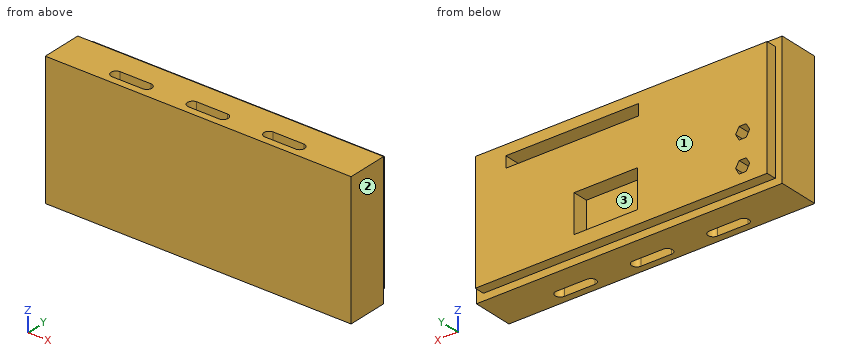
```python
from build123d import *

# Parameters (mm, degrees)
SKETCH1_W           = 150
SKETCH1_H           = 65
BOSS_EXTRUDE1_DEPTH = 20
CUT_EXTRUDE1_DEPTH  = 66
SKETCH3_W           = 143.142
SKETCH3_H           = 58.142
BOSS_EXTRUDE2_DEPTH = 5
CUT_EXTRUDE2_DEPTH  = 6.5
SKETCH6_W           = 65
SKETCH6_H           = 5.5
CUT_EXTRUDE3_DEPTH  = 10
SKETCH7_W           = 31
SKETCH7_H           = 18.5
CUT_EXTRUDE4_DEPTH  = 7.5


with BuildPart() as part:
    # Sketch1 → Boss-Extrude1 (new body)
    with BuildSketch(Plane(origin=(0, 0, 0), x_dir=(1, 0, 0), z_dir=(0, 1, 0))):
        Rectangle(SKETCH1_W, SKETCH1_H)
    extrude(amount=BOSS_EXTRUDE1_DEPTH)

    # Sketch2 → Cut-Extrude1 (cut, through all)
    with BuildSketch(Plane.XY.offset(32.5)):
        with BuildLine():
            Line((-7.5, 8.5), (7.5, 8.5))
            ThreePointArc((7.5, 8.5), (10, 6), (7.5, 3.5))
            Line((7.5, 3.5), (-7.5, 3.5))
            ThreePointArc((-7.5, 3.5), (-10, 6), (-7.5, 8.5))
        make_face()
        with BuildLine():
            Line((-45, 8.5), (-30, 8.5))
            ThreePointArc((-30, 8.5), (-27.5, 6), (-30, 3.5))
            Line((-30, 3.5), (-45, 3.5))
            ThreePointArc((-45, 3.5), (-47.5, 6), (-45, 8.5))
        make_face()
        with BuildLine():
            Line((30, 8.5), (45, 8.5))
            ThreePointArc((45, 8.5), (47.5, 6), (45, 3.5))
            Line((45, 3.5), (30, 3.5))
            ThreePointArc((30, 3.5), (27.5, 6), (30, 8.5))
        make_face()
    extrude(amount=-CUT_EXTRUDE1_DEPTH, mode=Mode.SUBTRACT)

    # Sketch3 → Boss-Extrude2 (add)
    with BuildSketch(Plane(origin=(0, 20, 0), x_dir=(1, 0, 0), z_dir=(0, 1, 0))):
        Rectangle(SKETCH3_W, SKETCH3_H)
    extrude(amount=BOSS_EXTRUDE2_DEPTH)

    # Sketch4 → Cut-Extrude2 (cut)
    with BuildSketch(Plane(origin=(0, 25, 0), x_dir=(1, 0, 0), z_dir=(0, 1, 0))):
        Polygon((-61.303050808, 24.571), (-63.035101615, 21.571), (-61.303050808, 18.571), (-57.838949192, 18.571), (-56.106898385, 21.571), (-57.838949192, 24.571), align=None)
        Polygon((-61.303050808, 9.551), (-63.035101615, 6.551), (-61.303050808, 3.551), (-57.838949192, 3.551), (-56.106898385, 6.551), (-57.838949192, 9.551), align=None)
    extrude(amount=-CUT_EXTRUDE2_DEPTH, mode=Mode.SUBTRACT)

    # Sketch6 → Cut-Extrude3 (cut)
    with BuildSketch(Plane(origin=(0, 25, 0), x_dir=(1, 0, 0), z_dir=(0, 1, 0))):
        with Locations((24.071, -21.321)):
            Rectangle(SKETCH6_W, SKETCH6_H)
    extrude(amount=-CUT_EXTRUDE3_DEPTH, mode=Mode.SUBTRACT)

    # Sketch7 → Cut-Extrude4 (cut)
    with BuildSketch(Plane(origin=(0, 25, 0), x_dir=(1, 0, 0), z_dir=(0, 1, 0))):
        with Locations((7.571, 13.321)):
            Rectangle(SKETCH7_W, SKETCH7_H)
    extrude(amount=-CUT_EXTRUDE4_DEPTH, mode=Mode.SUBTRACT)


solid = part.part
```
The model under review builds one solid part; all positions refer to its coordinate system, in mm. Face numbers are marked on the shaded views. Give positions to 0.01 mm unless a question says otherwise; leave off trailing zeros. Write each loop counter-clockwise with the first axis right and the second up, starting at its lowest first coordinate (ties: lowest second). Pieces come first, ordered by that corner, then holes. Notation, with made-up numbers: (62.25, -13.75) - (83.25, -13.75) arc R20 cw to (83.25, 20.25) - close; hole circle Ø1 at (62, 69). An arc over 180 degrees is marked (long way). Answer in a Markdown table with one row per item. Add a question column.
1. We need section D-D on x = 49.5. Write out the cut boundary in (y, z), then the cut area to 3 significant figures.
2. Wall thickness on line 1 along X through (y, z) = (6, 30); line 2 along Z through (x, y) = (51.5, 22); line 3 along Y through (x, z) = (-38, -8): over which ranges is each line inside the solid? List them lowest first. Write a range as [from, to].
3. We need section A-A on y = 6. Write out the cut boundary in (x, z).
4. We need section C-C on z = 11. Write out the cut boundary in (x, y).
5. Insertion check: P1, Ø6, axis at x = -33, y = 22.5, coming from the -Z side; P2, Ø3, axis at y = 22, z = 22, coming from the -X side; P3, Ø4, axis at x = 18, y = 22.5, coming from the +Z side; P4, Ø2, axis at y = 22, z = 14.5, coming from the +X side. Each pin has a flat end and moves straight along its axis. Give the tip position at first contact, or say it passes through.
6. We need section B-B on x = -3. Write out the cut boundary in (y, z), then the cut area to 3 significant figures.
7. Draft analysis for pull direction X (two halves, no side actions). For the marked faces 1, 2 and 3, state which applies: +X half, -X half, draft (parallel to the pull), parting line (faces both ways), or undercut.
Ans:
| question | item | result |
|---|---|---|
| 1 | outline | (0, -32.5) - (20, -32.5) - (20, -29.07) - (25, -29.07) - (25, 18.57) - (15, 18.57) - (15, 24.07) - (25, 24.07) - (25, 29.07) - (20, 29.07) - (20, 32.5) - (0, 32.5) - close |
| 1 | area | 1,540 mm^2 |
| 2 | line 1 | x = [-75, -47.5], [-27.5, -10], [10, 27.5], [47.5, 75] |
| 2 | line 2 | z = [-29.07, 18.57], [24.07, 29.07] |
| 2 | line 3 | y = [0, 3.5], [8.5, 25] |
| 3 | outline | (-75, -32.5) - (-47.5, -32.5) - (-47.5, 32.5) - (-75, 32.5) - close; (-27.5, -32.5) - (-10, -32.5) - (-10, 32.5) - (-27.5, 32.5) - close; (10, -32.5) - (27.5, -32.5) - (27.5, 32.5) - (10, 32.5) - close; (47.5, -32.5) - (75, -32.5) - (75, 32.5) - (47.5, 32.5) - close |
| 4 | outline | (-75, 0) - (75, 0) - (75, 20) - (71.57, 20) - (71.57, 25) - (-71.57, 25) - (-71.57, 20) - (-75, 20) - close; hole (-45, 3.5) - (-30, 3.5) arc R2.5 ccw to (-30, 8.5) - (-45, 8.5) arc R2.5 ccw to start; hole (-7.5, 3.5) - (7.5, 3.5) arc R2.5 ccw to (7.5, 8.5) - (-7.5, 8.5) arc R2.5 ccw to start; hole (30, 3.5) - (45, 3.5) arc R2.5 ccw to (45, 8.5) - (30, 8.5) arc R2.5 ccw to start |
| 5 | P1 | stops at z = -32.5 |
| 5 | P2 | stops at x = -71.57 |
| 5 | P3 | stops at z = 29.07 |
| 5 | P4 | stops at x = 71.57 |
| 6 | outline | (0, -32.5) - (3.5, -32.5) - (3.5, 32.5) - (0, 32.5) - close; (8.5, -32.5) - (20, -32.5) - (20, -29.07) - (25, -29.07) - (25, -22.57) - (17.5, -22.57) - (17.5, -4.07) - (25, -4.07) - (25, 18.57) - (15, 18.57) - (15, 24.07) - (25, 24.07) - (25, 29.07) - (20, 29.07) - (20, 32.5) - (8.5, 32.5) - close |
| 6 | area | 1,070 mm^2 |
| 7 | face 1 | draft |
| 7 | face 2 | +X half |
| 7 | face 3 | undercut |
